Part model, mm, in its own coordinate system. Face numbers are marked on the shaded views. A direction names the side the tool comes from. Give positions to 0.01 mm unless a question says otherwise; leave off trailing zeros. Order: outer loops, then holes, each group sorted by start corner. A loop starts at its lowest first (then second) coordinate and runs counter-clockwise, first axis right, second up. Notation, with made-up numbers: (33.25, -10) -> (84.25, -10) arc R26 ccw to (84.25, 9) -> close; hole circle Ø5 at (28, -5.75). An arc over 180 degrees is marked (long way). Write item = value, one per line. Start each with the question number.
(1) Which spindle directions (+Z, -Z, +X, -X, +Y, -Y) get a long thin tool onto all of the face, cutting with end or side? Do the marked faces 1 and 2. Say none if no direction does.
(2) Saw through at C-C, the plane y = 6. List the corners of the cut face in (x, z).
(3) Saw through at B-B, the plane x = -12. List the corners of the cut face in (y, z).
(4) Flat gauge pins, fed straight in: pin 1 (13 mm diameter, centred on x = 0, z = 0, fed in from +Y); pin 2 (5 mm diameter, centred on x = -4, y = 10, fed in from -Z); pin 3 (2 mm diameter, centred on y = 3.5, z = 2, fed in from -X); pin 4 (4 mm diameter, centred on y = 5.5, z = -5.5, fed in from +X). Where does each tip first touch, or does it go through?
(5) Probe line 1 along Z through (x, y) = (0, 1.5); line 2 along X through (y, z) = (1.8, 0); line 3 along Y through (x, z) = (4.5, 20). List the from-to ranges inside material, lowest first. Write a range as from..to.
(6) Saw through at A-A, the plane x = 0. List the corners of the cut face in (y, z).
(7) Saw through at D-D, the plane z = 12. List the corners of the cut face in (x, y).
from build123d import *

# Parameters (mm, degrees)
BOSS_EXTRUDE1_DEPTH = 3
SKETCH2_R           = 4
CUT_EXTRUDE1_DEPTH  = 13
BOSS_EXTRUDE2_DEPTH = 15.5


with BuildPart() as part:
    # Sketch1 → Boss-Extrude1 (new body)
    with BuildSketch(Plane(origin=(0, 0, 0), x_dir=(1, 0, 0), z_dir=(0, 1, 0))):
        with BuildLine():
            Line((-10, 0), (-14, -25))
            Line((-14, -25), (14, -25))
            Line((14, -25), (10, 0))
            ThreePointArc((10, 0), (0, 10), (-10, 0))
        make_face()
    extrude(amount=BOSS_EXTRUDE1_DEPTH)

    # Sketch2 → Cut-Extrude1 (cut)
    with BuildSketch(Plane(origin=(0, 3, 0), x_dir=(1, 0, 0), z_dir=(0, 1, 0))):
        Circle(SKETCH2_R)
    extrude(amount=-CUT_EXTRUDE1_DEPTH, mode=Mode.SUBTRACT)

    # Sketch5 → Boss-Extrude2 (add)
    with BuildSketch(Plane(origin=(0, 3, 0), x_dir=(1, 0, 0), z_dir=(0, 1, 0))):
        Polygon((-13.52, -22), (13.52, -22), (14, -25), (-14, -25), align=None)
    extrude(amount=BOSS_EXTRUDE2_DEPTH)


solid = part.part
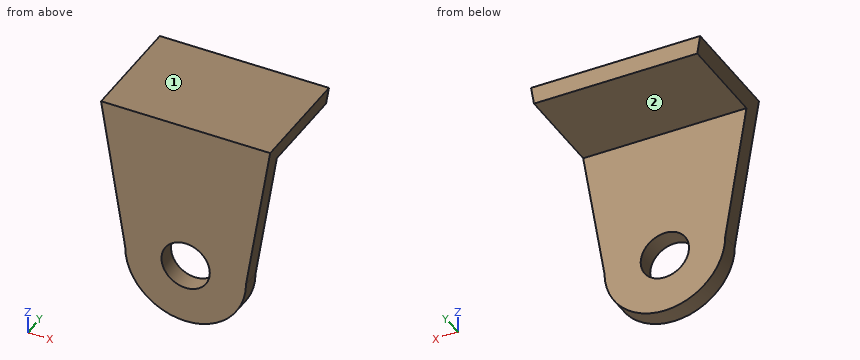
Results list:
q1.face_1 = +Z, +X, -X, +Y, -Y
q1.face_2 = -Z, +X, -X, +Y
q2.outline = (-14, 25) -> (-13.52, 22) -> (13.52, 22) -> (14, 25) -> close
q3.outline = (0, 12.5) -> (3, 12.5) -> (3, 22) -> (18.5, 22) -> (18.5, 25) -> (0, 25) -> close
q4.pin_1 = 3
q4.pin_2 = 22
q4.pin_3 = -10.46
q4.pin_4 = through
q5.line_1 = -10..-4, 4..25
q5.line_2 = -10..-4, 4..10
q5.line_3 = 0..3
q6.outline = (0, -10) -> (3, -10) -> (3, -4) -> (0, -4) -> close; (0, 4) -> (3, 4) -> (3, 22) -> (18.5, 22) -> (18.5, 25) -> (0, 25) -> close
q7.outline = (-11.92, 0) -> (11.92, 0) -> (11.92, 3) -> (-11.92, 3) -> close
